The figure shows three views and two pictorial views of one solid part (mm, origin at its lowest corner). Answer the questions. A direction names the side the tool comes from. Coordinates: 2 decimals unless noted, no trailing zeros. Write each loop counter-clockwise with the first axis right and the second up, starting at its lowest first coordinate (ties: lowest second). Pieces come first, ordered by that corner, then holes. Notation, with made-up numbers: M -9,8.25 L -1,8.25 A27 cw -1,44.25 Z; hole C -23,12.5 d6. An arc over 180 degrees is marked long. Write item = value, one per line.
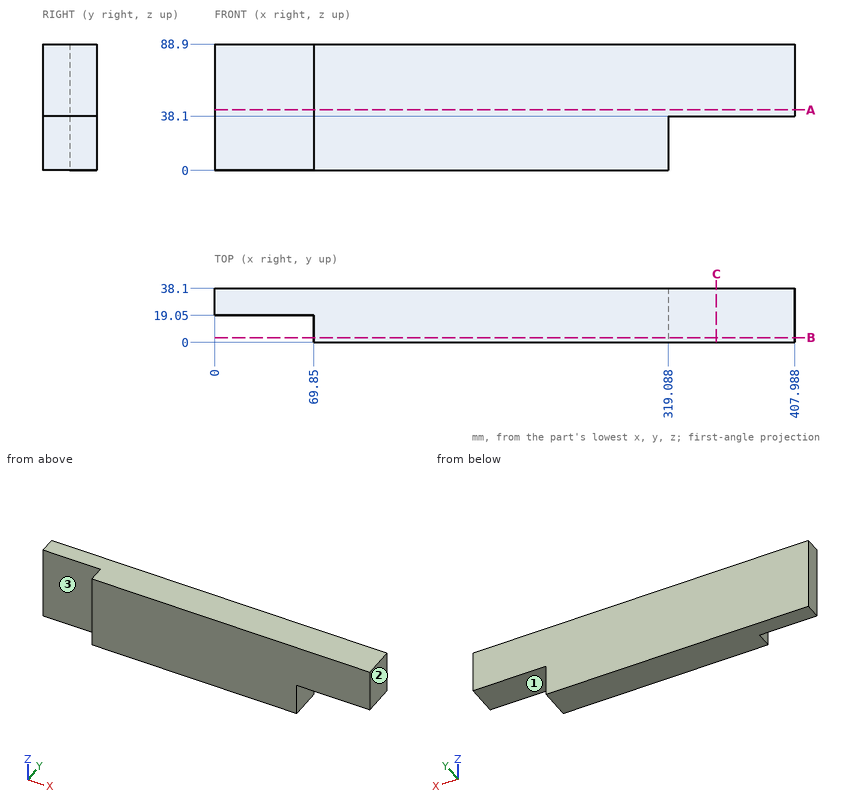
Item 1: Find section B-B (y = 3.5). Determine the outline of the cut face in (x, z), and give its area (3 significant figures).
Worked answers:
outline = M 69.85,0 L 319.09,0 L 319.09,38.1 L 407.99,38.1 L 407.99,88.9 L 69.85,88.9 Z
area = 26,700 mm²
Item 2: Find section A-A (z = 42.5). Determine the outline of the cut face in (x, y), and give its area (3 significant figures).
Worked answers:
outline = M 0,19.05 L 69.85,19.05 L 69.85,0 L 407.99,0 L 407.99,38.1 L 0,38.1 Z
area = 14,200 mm²
Item 3: Consider line 1 along X through (y, z) = (10, 11); line 2 along Z through (x, y) = (323.5, 11.5); line 3 along X through (y, z) = (4, 59). Determine where each line is inside the solid, lowest interval first. Write a range as from..to.
Worked answers:
line_1 = 69.85..319.09
line_2 = 38.1..88.9
line_3 = 69.85..407.99
Item 4: Flat-ended cylindrical pins translate along their axes: pin 1 (1 mm diameter, centred on x = 56, z = 71, fed in from -Y); pin 2 (9.5 mm diameter, centred on y = 7, z = 25, fed in from -X). Find the tip coordinate at first contact, or state that the pin passes through.
Worked answers:
pin_1 = 19.05
pin_2 = 69.85
Item 5: Which of the six approach directions +Z, -Z, +X, -X, +Y, -Y give full straight-line access (tool end or side, diameter ignored) to the marked faces 1, 2 and 3?
Worked answers:
face_1 = -Z, +X, +Y, -Y
face_2 = +Z, -Z, +X, +Y, -Y
face_3 = +Z, -Z, -X, -Y
Item 6: Find section C-C (x = 353). Determine the outline of the cut face in (y, z).
Worked answers:
outline = M 0,38.1 L 38.1,38.1 L 38.1,88.9 L 0,88.9 Z
